Geometry: final body of the model. Coordinates: model frame, mm. A direction names the side the tool comes from. Coordinates: 2 decimals unless noted, no trailing zeros. Loops run counter-clockwise (first coordinate to the right, second up) from the corner with the lowest first, then second, coordinate; pieces in that order, holes last. Notation, with made-up numbers: M -27.75,70.25 L -2.75,70.25 A15 ccw -2.75,81.25 Z; hole C -6.75,23 d4. An arc over 180 degrees is marked long. Write item = value, one per line. Start each with the question number.
```python
from build123d import *

# Parameters (mm, degrees)
SKETCH1_R           = 3.2639
SKETCH1_R_2         = 14.2875
SKETCH1_R_3         = 2.6289
BOSS_EXTRUDE1_DEPTH = 6.35
CUT_EXTRUDE1_DEPTH  = 6.35
CUT_EXTRUDE2_DEPTH  = 157.455309971
FILLET1_R           = 6.35
FILLET2_R           = 6.35
FILLET3_R           = 3.175
FILLET4_R           = 6.35
FILLET5_R           = 3.175
FILLET6_R           = 3.175
FILLET7_R           = 12.7
FILLET8_R           = 6.35


with BuildPart() as part:
    # Sketch1 → Boss-Extrude1 (new body)
    with BuildSketch(Plane(origin=(0, 0, 0), x_dir=(0, 0, -1), z_dir=(1, 0, 0))):
        with BuildLine():
            Line((0, 0), (76.2, 0))
            Line((76.2, 0), (118.05161028, 30.203441414))
            ThreePointArc((118.05161028, 30.203441414), (127.79577467, 57.092282399), (106.340627785, 76.003527237))
            Line((106.340627785, 76.003527237), (3.257374761, 88.899923295))
            ThreePointArc((3.257374761, 88.899923295), (-29.445545679, 65.344858986), (-22.705011853, 25.609644583))
            Line((-22.705011853, 25.609644583), (0, 0))
        make_face()
        with Locations((38.1, 12.7)):
            Circle(SKETCH1_R, mode=Mode.SUBTRACT)
        with Locations((63.5, 12.7)):
            Circle(SKETCH1_R, mode=Mode.SUBTRACT)
        with Locations((103.1875, 50.8)):
            Circle(SKETCH1_R_2, mode=Mode.SUBTRACT)
        with Locations((5.803937203, 50.885123286)):
            Circle(SKETCH1_R_2, mode=Mode.SUBTRACT)
        with Locations((5.803937203, 76.285123286)):
            Circle(SKETCH1_R_3, mode=Mode.SUBTRACT)
        with Locations((5.803937203, 25.485123286)):
            Circle(SKETCH1_R_3, mode=Mode.SUBTRACT)
        with Locations((31.203937203, 50.885123286)):
            Circle(SKETCH1_R_3, mode=Mode.SUBTRACT)
        with Locations((-19.596062797, 50.885123286)):
            Circle(SKETCH1_R_3, mode=Mode.SUBTRACT)
    extrude(amount=BOSS_EXTRUDE1_DEPTH)

    # Sketch2 → Cut-Extrude1 (cut)
    with BuildSketch(Plane.ZY):
        Polygon((0, 0), (-25.4, 0), (-25.4, 12.7), (0, 12.7), (11.95076388, 12.7), (11.95076388, 0), align=None)
    extrude(amount=-CUT_EXTRUDE1_DEPTH, mode=Mode.SUBTRACT)

    # Sketch3 → Cut-Extrude2 (cut, through all)
    with BuildSketch(Plane.ZY):
        Polygon((-105.957463546, 25.4), (-43.903937203, 50.885123286), (-38.1, 25.4), align=None)
        Polygon((-88.713516137, 69.889443956), (-77.333414898, 50.885123286), (-5.803937203, 80.261980092), align=None)
    extrude(amount=-CUT_EXTRUDE2_DEPTH, mode=Mode.SUBTRACT)

    # Fillet1
    fillet1_edges = [part.edges().sort_by_distance(p)[0] for p in [
        (3.175, 50.885123286, -77.333414898),
    ]]
    fillet(fillet1_edges, radius=FILLET1_R)

    # Fillet2
    fillet2_edges = [part.edges().sort_by_distance(p)[0] for p in [
        (3.175, 69.889443956, -88.713516137),
    ]]
    fillet(fillet2_edges, radius=FILLET2_R)

    # Fillet3
    fillet3_edges = [part.edges().sort_by_distance(p)[0] for p in [
        (3.175, 80.261980092, -5.803937203),
    ]]
    fillet(fillet3_edges, radius=FILLET3_R)

    # Fillet4
    fillet4_edges = [part.edges().sort_by_distance(p)[0] for p in [
        (3.175, 50.885123286, -43.903937203),
    ]]
    fillet(fillet4_edges, radius=FILLET4_R)

    # Fillet5
    fillet5_edges = [part.edges().sort_by_distance(p)[0] for p in [
        (3.175, 25.4, -38.1),
    ]]
    fillet(fillet5_edges, radius=FILLET5_R)

    # Fillet6
    fillet6_edges = [part.edges().sort_by_distance(p)[0] for p in [
        (3.175, 25.4, -105.957463546),
    ]]
    fillet(fillet6_edges, radius=FILLET6_R)

    # Fillet7
    fillet7_edges = [part.edges().sort_by_distance(p)[0] for p in [
        (3.175, 12.7, -25.4),
    ]]
    fillet(fillet7_edges, radius=FILLET7_R - 0.0001)  # a hair under: the kernel refuses the full size

    # Fillet8
    fillet8_edges = [part.edges().sort_by_distance(p)[0] for p in [
        (3.175, 12.7, 11.259572526),
    ]]
    fillet(fillet8_edges, radius=FILLET8_R)


solid = part.part
```
Item 1: First-contact query: pin 1 (2 mm diameter, centred on x = 1, z = -48.5, fed in from +Y); pin 2 (3 mm diameter, centred on x = 4, z = -5, fed in from -Y); pin 3 (3 mm diameter, centred on x = 1, z = -95, fed in from +Y); pin 4 (6 mm diameter, centred on y = 12.7, z = -38.1, fed in from -X). Flat tips, straight axial feed; report the tip coordinate or a pass-through.
Item 2: Section query D-D (z = -17). Return the cut outline in (x, y), plus the area to 3 significant figures.
Item 3: Section query A-A (z = -63.5). Return the cut outline in (x, y).
Item 4: Section query C-C (x = 5). Count the separate pieces of the cut face and the enclosed holes in it, plus the area to 3 significant figures.
Item 5: Pull-direction query (Y, two-part tool) for faces 1 (the flat face through (3.13, 82.36, -55.52)), 2 (the flat face through (6.35, 55, -47)), 3 (the flat face through (3, 12.7, -2)), 4 (the cylindrical face through (3.22, 27.9, -92.97)); classes: released by +Y, released by -Y, zero draft, split by the parting line, or undercut.
Item 6: Section query B-B (y = 34.5). Return the cut outline in (x, z).
Item 7: Line query: line 1 (Y direction, x = 4.25, z = -66.5); line 2 (Y direction, x = 5.5, z = -47); line 3 (Y direction, x = 3.5, z = -63.5). Output: solid intervals per line, ascending. Write a range as from..to.
Item 8: Reachability of faces 5 (the flat face through (3, 0, -50)), 6 (the cylindrical face through (3.219, 75.026, -25.973)) from +Z, -Z, +X, -X, +Y, -Y: full face, straight path, thin tool, end or side. Return the list, or none.
Verdict:
q1.pin_1 = 83.36
q1.pin_2 = 12.7
q1.pin_3 = 77.61
q1.pin_4 = through
q2.outline = M 0,11.95 L 6.35,11.95 L 6.35,42.01 L 0,42.01 Z; M 0,59.76 L 6.35,59.76 L 6.35,87.18 L 0,87.18 Z
q2.area = 365 mm2
q3.outline = M 0,0 L 6.35,0 L 6.35,9.44 L 0,9.44 Z; M 0,15.96 L 6.35,15.96 L 6.35,25.4 L 0,25.4 Z; M 0,42.84 L 6.35,42.84 L 6.35,56.57 L 0,56.57 Z; M 0,73.04 L 6.35,73.04 L 6.35,81.36 L 0,81.36 Z
q4.separate_pieces = 1
q4.enclosed_holes = 10
q4.area = 7,910 mm2
q5.face_1 = released by +Y
q5.face_2 = zero draft
q5.face_3 = released by -Y
q5.face_4 = undercut
q6.outline = M 0,-122.67 L 6.35,-122.67 L 6.35,-83.8 L 0,-83.8 Z; M 0,-40.17 L 6.35,-40.17 L 6.35,28.59 L 0,28.59 Z
q7.line_1 = 0..11.41, 13.99..25.4, 41.61..55.33, 72.67..80.99
q7.line_2 = 0..25.4, 48.35..63.34, 75.11..83.43
q7.line_3 = 0..9.44, 15.96..25.4, 42.84..56.57, 73.04..81.36
q8.face_5 = +Z, -Z, +X, -X, -Y
q8.face_6 = +X, -X
